The listing builds one solid part. Answer for the finished solid, in the listing's coordinates (mm). Face numbers are marked on the shaded views. Round coordinates to 2 decimals unless told otherwise and drop trailing zeros. Write each loop counter-clockwise with the first axis right and the second up, starting at its lowest first coordinate (ties: lowest second). Pieces come first, ordered by that corner, then holes. Notation, with made-up numbers: (84, 50) - (121, 50) arc R24 cw to (121, 80) - close; hole circle Ø9 at (38, -22). An arc over 180 degrees is marked (long way). Answer in a Markdown table with one row per item.
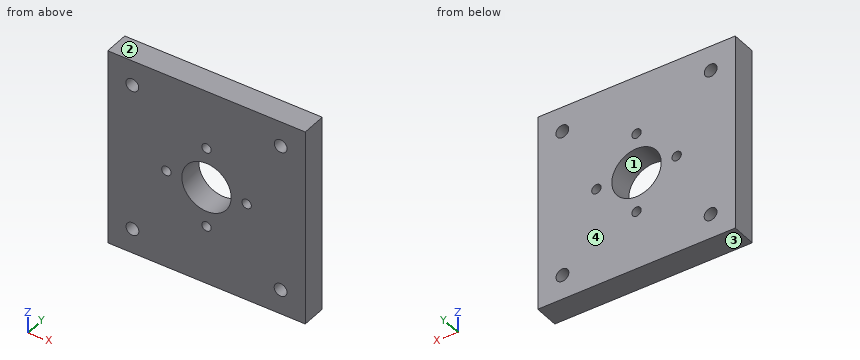
from build123d import *

# Parameters (mm, degrees)
SKETCH2_W           = 101.6
SKETCH2_H           = 101.6
BOSS_EXTRUDE1_DEPTH = 12.7
SKETCH3_R           = 3.302
CUT_EXTRUDE1_DEPTH  = 12.7
SKETCH4_R           = 12.7
CUT_EXTRUDE2_DEPTH  = 12.7
SKETCH5_R           = 2.413
CUT_EXTRUDE3_DEPTH  = 63.5


with BuildPart() as part:
    # Sketch2 → Boss-Extrude1 (new body)
    with BuildSketch(Plane(origin=(0, 0, 0), x_dir=(1, 0, 0), z_dir=(0, 1, 0))):
        Rectangle(SKETCH2_W, SKETCH2_H)
    extrude(amount=BOSS_EXTRUDE1_DEPTH)

    # Sketch3 → Cut-Extrude1 (cut)
    with BuildSketch(Plane(origin=(0, 12.7, 0), x_dir=(1, 0, 0), z_dir=(0, 1, 0))):
        with Locations(Location((-38.1, 38.1, 0), (0, 0, 270))):
            Circle(SKETCH3_R)
        with Locations(Location((-38.15484628, -37.971770083, 0), (0, 0, 90))):
            Circle(SKETCH3_R)
        with Locations(Location((38.15484628, -37.971770083, 0), (0, 0, 270))):
            Circle(SKETCH3_R)
        with Locations(Location((38.1, 38.1, 0), (0, 0, 90))):
            Circle(SKETCH3_R)
    extrude(amount=-CUT_EXTRUDE1_DEPTH, mode=Mode.SUBTRACT)

    # Sketch4 → Cut-Extrude2 (cut)
    with BuildSketch(Plane(origin=(0, 12.7, 0), x_dir=(1, 0, 0), z_dir=(0, 1, 0))):
        with Locations(Location((0, 0, 0), (0, 0, 270))):
            Circle(SKETCH4_R)
    extrude(amount=-CUT_EXTRUDE2_DEPTH, mode=Mode.SUBTRACT)

    # Sketch5 → Cut-Extrude3 (cut)
    with BuildSketch(Plane(origin=(0, 12.7, 0), x_dir=(1, 0, 0), z_dir=(0, 1, 0))):
        with Locations(Location((0, 20.6375, 0), (0, 0, 270))):
            Circle(SKETCH5_R)
        with Locations(Location((20.6375, 0, 0), (0, 0, 270))):
            Circle(SKETCH5_R)
        with Locations(Location((0, -20.6375, 0), (0, 0, 270))):
            Circle(SKETCH5_R)
        with Locations(Location((-20.6375, 0, 0), (0, 0, 270))):
            Circle(SKETCH5_R)
    extrude(amount=-CUT_EXTRUDE3_DEPTH, mode=Mode.SUBTRACT)


solid = part.part
(1) For a pull along Z with two mould halves and no side action, classify the marked faces 1, 2, 3 and 4 as pulls with the +Z half, pulls with the -Z half, needs draft (parallel to the pull), parting line crosses it, or undercut.
Checked values:
| item | result |
|---|---|
| face 1 | undercut |
| face 2 | pulls with the +Z half |
| face 3 | pulls with the -Z half |
| face 4 | needs draft |
(2) A flat-ended cylindrical pin translates along its axis: pin 1 (6.5 mm diameter, centred on x = 20.64, z = 0, fed in from +Y). Find the tip coordinate at first contact, or state that the pin passes through.
Checked values:
| item | result |
|---|---|
| pin 1 | stops at y = 12.7 |
(3) Section C-C (z = 40) is taken. Give the vertices of the cut face in (x, y), and give its area (3 significant figures).
Checked values:
| item | result |
|---|---|
| outline | (-50.8, 0) - (-40.76, 0) - (-40.76, 12.7) - (-50.8, 12.7) - close; (-35.55, 0) - (35.55, 0) - (35.55, 12.7) - (-35.55, 12.7) - close; (40.76, 0) - (50.8, 0) - (50.8, 12.7) - (40.76, 12.7) - close |
| area | 1,160 mm2 |
(4) Section A-A (z = 0) is taken. Give the vertices of the cut face in (x, y).
Checked values:
| item | result |
|---|---|
| outline | (-50.8, 0) - (-23.05, 0) - (-23.05, 12.7) - (-50.8, 12.7) - close; (-18.22, 0) - (-12.7, 0) - (-12.7, 12.7) - (-18.22, 12.7) - close; (12.7, 0) - (18.22, 0) - (18.22, 12.7) - (12.7, 12.7) - close; (23.05, 0) - (50.8, 0) - (50.8, 12.7) - (23.05, 12.7) - close |
(5) Section B-B (x = 0) is taken. Give the vertices of the cut face in (y, z), and give its area (3 significant figures).
Checked values:
| item | result |
|---|---|
| outline | (0, -50.8) - (12.7, -50.8) - (12.7, -23.05) - (0, -23.05) - close; (0, -18.22) - (12.7, -18.22) - (12.7, -12.7) - (0, -12.7) - close; (0, 12.7) - (12.7, 12.7) - (12.7, 18.22) - (0, 18.22) - close; (0, 23.05) - (12.7, 23.05) - (12.7, 50.8) - (0, 50.8) - close |
| area | 845 mm2 |
(6) Find the intervals of material crossed by line 1 (X direction, y = 9.5, z = -38.1); line 2 (X direction, y = 4.5, z = 0); line 3 (Z direction, x = -38, y = 7.5), in increasing order.
Checked values:
| item | result |
|---|---|
| line 1 | x = -50.8 to -41.4, -34.8 to 34.8, 41.4 to 50.8 |
| line 2 | x = -50.8 to -23.05, -18.22 to -12.7, 12.7 to 18.22, 23.05 to 50.8 |
| line 3 | z = -50.8 to -41.4, -34.8 to 34.67, 41.27 to 50.8 |
(7) Section D-D (y = 7.5) is taken. State how many separate pieces and enclosed holes the cut face has, and give its area (3 significant figures).
Checked values:
| item | result |
|---|---|
| separate pieces | 1 |
| enclosed holes | 9 |
| area | 9,610 mm2 |
